Input: part model. Units: mm. Frame: model coordinates. A direction names the side the tool comes from. Round coordinates to 2 decimals unless told otherwise and drop trailing zeros. Loops run counter-clockwise (first coordinate to the right, second up) from the corner with the lowest first, then second, coordinate; pieces in that order, holes last. Notation, with made-up numbers: M 28,64.5 L 78,64.5 A14 cw 78,90.5 Z; hole C 9.25,36 d2. An arc over 180 degrees is marked long. Return JSON: item names as keys, results as strings. Group by question number.
1) Mould query, pull axis Y, two halves, no side actions, for faces 4 (the face through (6, 8, 0)), 5 (the face through (-3.347, -48.722, -0.147)), 6 (the face through (0, -87, 0)). Classes: +Y half, -Y half, draft (parallel to the pull), parting line (faces both ways), or undercut.
2) Contact query for flat-ended pins moving along their axis: P1, Ø1.5, axis at y = 51.5, z = -1.5, coming from the -X side; P2, Ø1.5, axis at y = -1, z = 1, coming from the +X side; P3, Ø3, axis at x = -1.5, y = -23.5, coming from the -Z side. Output: stop coordinate, or through.
3) Section C-C (y = 49). Output: boundary loops of the cut face in (x, z).
4) Section A-A (x = 0). Output: boundary loops of the cut face in (y, z).
5) Access query for faces 1 (the face through (-6, 8, 0)), 2 (the face through (-3.347, 49.214, 0.147)), 3 (the face through (0, 103, 0)). Directions: +Z, -Z, +X, -X, +Y, -Y. A direction counts if a zero-diameter tool reaches every point of the face in a straight line with its end or side. Return the directions, or none.
6) Material intervals for line 1 (Y direction, x = 2, z = -2.5); line 2 (Y direction, x = 5.75, z = 0.75); line 3 (X direction, y = 18, z = 2.25), sorted ascending. Write a range as from..to.
7) Section B-B (z = 0). Output: boundary loops of the cut face in (x, y), plus the area to 3 significant figures.
Autodesk Inventor part; units mm, degrees
ref_plane "YZ Plane" through (0, 0, 0) normal (1, 0, 0) x (0, 1, 0)
ref_plane "XZ Plane" through (0, 0, 0) normal (0, 1, 0) x (-1, 0, 0)
ref_plane "XY Plane" through (0, 0, 0) normal (0, 0, 1) x (1, 0, 0)
sketch "Sketch1" plane through (0, 0, 0) normal (0, 1, 0) x (-1, 0, 0)
  line L0 (12.5, 0) -> (12.5, 4.5) construction
  line L1 (12.5, 4.5) -> (12.5, -4.5) construction
  line L2 (11.6619, 4.5) -> (-11.6619, 4.5)
  line L3 (11.6619, -4.5) -> (-11.6619, -4.5)
  arc A0 (11.6619, -4.5) -> (11.6619, 4.5) centre (0, 0) ccw
  arc A1 (-11.6619, 4.5) -> (-11.6619, -4.5) centre (0, 0) ccw
  dimension "d1" = 4.5
  dimension "d2" = 9
extrude "Extrusion1" add sketch "Sketch1" along normal mid plane 23
sketch "Sketch2" plane through (-11.6619, -11.5, 4.5) normal (0, 0, 1) x (1, 0, 0)
  line L0 (7.1619, 5) -> (16.1619, 5)
  line L1 (19.1619, 5) -> (19.1619, 18)
  line L2 (4.1619, 18) -> (4.1619, 5)
  line L3 (11.6619, 11.5) -> (19.1619, 18) construction
  line L4 (19.1619, 5) -> (11.6619, 11.5) construction
  line L5 (4.1619, 5) -> (5.6619, 5) construction
  arc A0 (4.1619, 5) -> (7.1619, 5) centre (5.6619, 5) ccw
  line L6 (4.1619, 18) -> (5.6619, 18) construction
  arc A1 (7.1619, 18) -> (4.1619, 18) centre (5.6619, 18) ccw
  line L7 (19.1619, 5) -> (17.6619, 5) construction
  arc A2 (16.1619, 5) -> (19.1619, 5) centre (17.6619, 5) ccw
  arc A3 (17.6619, 6.5) -> (17.4487, 6.4848) centre (17.6619, 5) ccw
  arc A4 (19.1619, 18) -> (16.1619, 18) centre (17.6619, 18) ccw
  arc A5 (17.4487, 16.5152) -> (17.6619, 16.5) centre (17.6619, 18) ccw
  line L8 (16.1619, 18) -> (7.1619, 18)
  dimension "d8" = 1.5
extrude "Extrusion2" cut sketch "Sketch2" against normal through all
sketch "Sketch3" plane through (0, -11.5, 0) normal (0, -1, 0) x (1, 0, 0)
  circle A0 centre (0, 0) radius 3.35
  dimension "d11" = 6.7
extrude "Extrusion3" add sketch "Sketch3" along normal blind 75.5
sketch "Sketch4" plane through (0, 11.5, 0) normal (0, 1, 0) x (1, 0, 0)
  circle A0 centre (0, 0) radius 3.35
  dimension "d14" = 6.7
extrude "Extrusion4" add sketch "Sketch4" along normal blind 76.5
sketch "Sketch5" plane through (0, 88, 0) normal (0, 1, 0) x (1, 0, 0)
  circle A0 centre (0, 0) radius 2.5
  dimension "d17" = 5
extrude "Extrusion5" add sketch "Sketch5" along normal blind 15
thread "Thread1"
properties part number "Asta pistone"
Returned:
{
 "1": {"face 4": "undercut", "face 5": "draft", "face 6": "-Y half"},
 "2": {"P1": "stops at x = -3.26", "P2": "stops at x = 12.5", "P3": "stops at z = -3.35"},
 "3": {"outline": "C 0,0 d6.7"},
 "4": {"outline": "M -87,-3.35 L -11.5,-3.35 L -11.5,-4.5 L -6.5,-4.5 L -6.5,4.5 L -11.5,4.5 L -11.5,3.35 L -87,3.35 Z; M 6.5,-4.5 L 11.5,-4.5 L 11.5,-3.35 L 88,-3.35 L 88,-2.5 L 103,-2.5 L 103,2.5 L 88,2.5 L 88,3.35 L 11.5,3.35 L 11.5,4.5 L 6.5,4.5 Z"},
 "5": {"face 1": "+Z, -Z", "face 2": "+Y", "face 3": "+Z, -Z, +X, -X, +Y"},
 "6": {"line 1": "y = -87..-6.5, 6.5..88", "line 2": "y = -11.5..-7.98, 7.98..11.5", "line 3": "x = -2.48..2.48"},
 "7": {"outline": "M -12.5,-11.5 L -3.35,-11.5 L -3.35,-87 L 3.35,-87 L 3.35,-11.5 L 12.5,-11.5 L 12.5,11.5 L 3.35,11.5 L 3.35,88 L 2.5,88 L 2.5,103 L -2.5,103 L -2.5,88 L -3.35,88 L -3.35,11.5 L -12.5,11.5 Z; hole M -7.5,-6.5 A1.5 ccw -4.5,-6.5 L 4.5,-6.5 A1.5 ccw 7.5,-6.5 L 7.5,6.5 A1.5 ccw 4.5,6.5 L -4.5,6.5 A1.5 ccw -7.5,6.5 Z", "area": "1,460 mm^2"}
}
